CAD build for the part. Positions are in the model's coordinates, mm. Round coordinates to 2 decimals unless told otherwise and drop trailing zeros. Loops run counter-clockwise (first coordinate to the right, second up) from the corner with the lowest first, then second, coordinate; pieces in that order, holes last. Notation, with made-up numbers: (-38.75, 40) - (5.25, 40) arc R16 cw to (5.25, 70) - close; hole circle Ø10 at (34, -20.75). An arc over 180 degrees is marked (long way). Use one line per item in the form item = value.
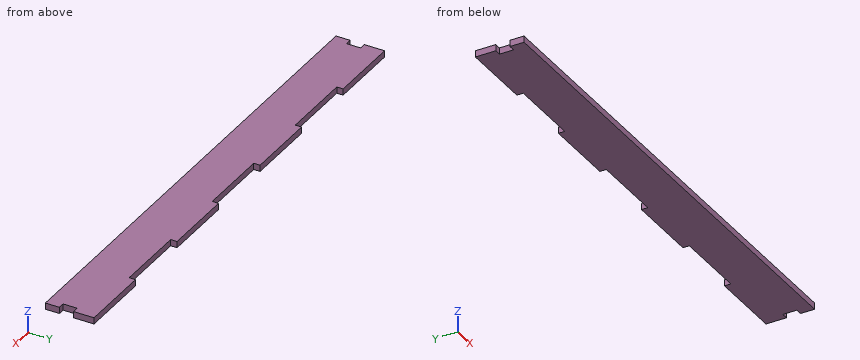
from build123d import *

# Parameters (mm, degrees)
SKETCH1_W               = 466
SKETCH1_H               = 126.5
BOSS_EXTRUDE1_DEPTH     = 6
SKETCH2_W               = 68.285714285
SKETCH2_H               = 6
SKETCH2_W_2             = 68.285714286
BOSS_EXTRUDE2_DEPTH     = 40
SKETCH1_2_W             = 466
SKETCH1_2_H             = 126.5
CUT_EXTRUDE1_DEPTH      = 7
CUT_EXTRUDE1_DEPTH_BACK = 35
SKETCH2_4_W             = 68.285714286
SKETCH2_4_H             = 6
BOSS_EXTRUDE3_DEPTH     = 6
SKETCH3_W               = 6
SKETCH3_H               = 13.333333334
CUT_EXTRUDE2_DEPTH      = 6


with BuildPart() as part:
    # Sketch1 → Boss-Extrude1 (new body)
    with BuildSketch(Plane(origin=(0, 0, 0), x_dir=(1, 0, 0), z_dir=(0, 1, 0))):
        Rectangle(SKETCH1_W, SKETCH1_H)
    extrude(amount=BOSS_EXTRUDE1_DEPTH)

    # Sketch2 → Boss-Extrude2 (add)
    with BuildSketch(Plane(origin=(0, 6, 0), x_dir=(1, 0, 0), z_dir=(0, 1, 0))):
        Polygon((-239, 69.25), (-239, 63.25), (-233, 63.25), (-170.714285714, 63.25), (-170.714285714, 69.25), align=None)
        with Locations((-136.571428572, 66.25)):
            Rectangle(SKETCH2_W, SKETCH2_H)
        with Locations((-68.285714286, 66.25)):
            Rectangle(SKETCH2_W_2, SKETCH2_H)
        with Locations((0, 66.25)):
            Rectangle(SKETCH2_W_2, SKETCH2_H)
        with Locations((68.285714286, 66.25)):
            Rectangle(SKETCH2_W_2, SKETCH2_H)
        with Locations((136.571428572, 66.25)):
            Rectangle(SKETCH2_W, SKETCH2_H)
        Polygon((233, 63.25), (239, 63.25), (239, 69.25), (170.714285714, 69.25), (170.714285714, 63.25), align=None)
    extrude(amount=-BOSS_EXTRUDE2_DEPTH)

    # Sketch1<2> → Cut-Extrude1 (cut, two sides)
    with BuildSketch(Plane(origin=(0, 0, 0), x_dir=(1, 0, 0), z_dir=(0, 1, 0))) as cut_extrude1_sk:
        Rectangle(SKETCH1_2_W, SKETCH1_2_H)
    extrude(amount=CUT_EXTRUDE1_DEPTH, mode=Mode.SUBTRACT)
    extrude(cut_extrude1_sk.sketch, amount=-CUT_EXTRUDE1_DEPTH_BACK, mode=Mode.SUBTRACT)

    # Sketch2<4> → Boss-Extrude3 (add)
    with BuildSketch(Plane(origin=(0, 6, 0), x_dir=(1, 0, 0), z_dir=(0, 1, 0))):
        Polygon((-239, 69.25), (-239, 63.25), (-233, 63.25), (-170.714285714, 63.25), (-170.714285714, 69.25), align=None)
        with Locations((-68.285714286, 66.25)):
            Rectangle(SKETCH2_4_W, SKETCH2_4_H)
        with Locations((68.285714286, 66.25)):
            Rectangle(SKETCH2_4_W, SKETCH2_4_H)
        Polygon((233, 63.25), (239, 63.25), (239, 69.25), (170.714285714, 69.25), (170.714285714, 63.25), align=None)
    extrude(amount=BOSS_EXTRUDE3_DEPTH)

    # Sketch3 → Cut-Extrude2 (cut)
    with BuildSketch(Plane.XY.offset(-63.25)):
        with Locations((-236, -14)):
            Rectangle(SKETCH3_W, SKETCH3_H)
    cut_extrude2 = extrude(amount=-CUT_EXTRUDE2_DEPTH, mode=Mode.SUBTRACT)

    # Mirror1: Cut-Extrude2 across plane
    add(cut_extrude2.mirror(Plane(origin=(0, 0, 0), x_dir=(0, 0, 1), z_dir=(1, 0, 0))), mode=Mode.SUBTRACT)


solid = part.part
1) Flat gauge pins, fed straight in: pin 1 (1 mm diameter, centred on y = -18, z = -66, fed in from -X); pin 2 (1.8 mm diameter, centred on x = -3, z = -65.5, fed in from +Y). Where does each tip first touch, or does it go through?
Report:
pin_1 = -233
pin_2 = 6
2) Slice it at B-B (x = -29). Write the cut outline in (y, z).
Report:
outline = (-34, -69.25) - (6, -69.25) - (6, -63.25) - (-34, -63.25) - close
3) Drill centre lines: probe 1 along X at (y, z) = (10.5, -67.75); probe 2 along X at (y, z) = (-12, -67.4); probe 3 along Y at (x, z) = (-31.5, -67.4). Where is each one in solid material? Low to high.
Report:
probe_1 = -239 to -170.71, -102.43 to -34.14, 34.14 to 102.43, 170.71 to 239
probe_2 = -233 to 233
probe_3 = -34 to 6
4) Slice it at A-A (z = -67). Write the cut outline in (x, y).
Report:
outline = (-239, -34) - (239, -34) - (239, -20.67) - (233, -20.67) - (233, -7.33) - (239, -7.33) - (239, 12) - (170.71, 12) - (170.71, 6) - (102.43, 6) - (102.43, 12) - (34.14, 12) - (34.14, 6) - (-34.14, 6) - (-34.14, 12) - (-102.43, 12) - (-102.43, 6) - (-170.71, 6) - (-170.71, 12) - (-239, 12) - (-239, -7.33) - (-233, -7.33) - (-233, -20.67) - (-239, -20.67) - close
